```python
from build123d import *

# Parameters (mm, degrees)
BOSS_EXTRUDE1_DEPTH = 340
SKETCH3_R           = 10
CUT_EXTRUDE1_DEPTH  = 340
SKETCH4_R           = 3
CUT_EXTRUDE2_DEPTH  = 25


with BuildPart() as part:
    # Sketch2 → Boss-Extrude1 (new body)
    with BuildSketch(Plane.XY):
        Polygon((0, 0), (24, 0), (24, -1), (1, -1), (1, -44), (24, -44), (24, -45), (0, -45), align=None)
    extrude(amount=BOSS_EXTRUDE1_DEPTH)

    # Sketch3 → Cut-Extrude1 (cut)
    with BuildSketch(Plane.ZY):
        with Locations((30, -22.5)):
            Circle(SKETCH3_R)
        with Locations((310, -22.5)):
            Circle(SKETCH3_R)
    extrude(amount=-CUT_EXTRUDE1_DEPTH, mode=Mode.SUBTRACT)

    # Sketch4 → Cut-Extrude2 (cut)
    with BuildSketch(Plane(origin=(0, 0, 0), x_dir=(1, 0, 0), z_dir=(0, 1, 0))):
        with Locations((12, -170)):
            Circle(SKETCH4_R)
    extrude(amount=-CUT_EXTRUDE2_DEPTH, mode=Mode.SUBTRACT)


solid = part.part
```
The listing builds one solid part. Answer for the finished solid, in the listing's coordinates (mm). A direction names the side the tool comes from. Coordinates: 2 decimals unless noted, no trailing zeros. Loops run counter-clockwise (first coordinate to the right, second up) from the corner with the lowest first, then second, coordinate; pieces in that order, holes last. Notation, with made-up numbers: (-9.75, -6.75) - (-2.75, -6.75) arc R36 ccw to (-2.75, 32.25) - close; hole circle Ø8 at (41, -9). An arc over 180 degrees is marked (long way). Use a Markdown table: item, result. Add a question column.
1) The part is cut by section D-D, the plane z = 98. Give the vertices of the cut face in (x, y).
2) The part is cut by section C-C, the plane x = 12. Give the vertices of the cut face in (y, z).
3) The part is cut by section A-A, the plane y = -22.5. Give the vertices of the cut face in (x, z), and give its area (3 significant figures).
4) Given pin 1 (10 mm diameter, centred on y = -28.5, z = 198, fed in from +X), flat-ended and moving along its own axis, determine where the tip first touches the part or whether it passes through.
5) The part is cut by section B-B, the plane z = 170. Give the vertices of the cut face in (x, y).
6) For faces 1 (the cylindrical face through (11.609, -0.493, 167.026)), 2 (the flat face through (1, -22, 168)), 3 (the cylindrical face through (0.49, -19.5, 39.54)), determine the directions among +Z, -Z, +X, -X, +Y, -Y from which every point of the face is accessible in a straight line to the end or side of a thin tool.
7) Find the intervals of material crossed by line 1 (Y direction, x = 10.75, z = 20); line 2 (Y direction, x = 0.4, z = 30); line 3 (X direction, y = -0.4, z = 170), in increasing order.
8) The mould has two halves that part along Y. Classify faces 4 (the flat face through (15, -1, 168)), 5 (the flat face through (0.5, -22.4, 0)), 6 (the flat face through (9, 0, 168)), 7 (the flat face through (12, -45, 168)): released by +Y, released by -Y, zero draft, split by the parting line, or undercut.
Here are the results:
| question | item | result |
|---|---|---|
| 1 | outline | (0, -45) - (24, -45) - (24, -44) - (1, -44) - (1, -1) - (24, -1) - (24, 0) - (0, 0) - close |
| 2 | outline | (-45, 0) - (-44, 0) - (-44, 340) - (-45, 340) - close; (-1, 0) - (0, 0) - (0, 167) - (-1, 167) - close; (-1, 173) - (0, 173) - (0, 340) - (-1, 340) - close |
| 3 | outline | (0, 0) - (1, 0) - (1, 20) - (0, 20) - close; (0, 40) - (1, 40) - (1, 300) - (0, 300) - close; (0, 320) - (1, 320) - (1, 340) - (0, 340) - close |
| 3 | area | 300 mm^2 |
| 4 | pin 1 | stops at x = 1 |
| 5 | outline | (0, -45) - (24, -45) - (24, -44) - (1, -44) - (1, -1) - (9, -1) - (9, 0) - (0, 0) - close; (15, -1) - (24, -1) - (24, 0) - (15, 0) - close |
| 6 | face 1 | +Y |
| 6 | face 2 | +Z, -Z, +X |
| 6 | face 3 | +X, -X |
| 7 | line 1 | y = -45 to -44, -1 to 0 |
| 7 | line 2 | y = -45 to -32.5, -12.5 to 0 |
| 7 | line 3 | x = 0 to 9, 15 to 24 |
| 8 | face 4 | undercut |
| 8 | face 5 | zero draft |
| 8 | face 6 | released by +Y |
| 8 | face 7 | released by -Y |
